```python
from build123d import *

# Parameters (mm, degrees)
F1_DEPTH = 150
F2_R     = 10
F4_W     = 30
F4_H     = 20
F5_DEPTH = 25
F6_R     = 7.5
F7_DEPTH = 10
F8_DEPTH = 25


with BuildPart() as f1:
    # F0 (on Top) → F1 (new body)
    with BuildSketch(Plane.XY):
        Polygon((0, 50), (-47.5528258148, 15.4508497187), (-29.3892626146, -40.4508497187), (29.3892626146, -40.4508497187), (47.5528258148, 15.4508497187), align=None)
    extrude(amount=F1_DEPTH)

    # F2
    f2_edges = [f1.edges().sort_by_distance(p)[0] for p in [
        (-29.389263, -40.45085, 75),
        (-47.552826, 15.45085, 75),
        (0, 50, 75),
        (47.552826, 15.45085, 75),
        (29.389263, -40.45085, 75),
    ]]
    fillet(f2_edges, radius=F2_R)

    # F4 (on face) → F5 (cut)
    with BuildSketch(Plane.XY.offset(150)):
        Rectangle(F4_W, F4_H)
    extrude(amount=-F5_DEPTH, mode=Mode.SUBTRACT)

    # F6 (on face) → F7 (cut)
    with BuildSketch(Plane.XZ.offset(40.4508497187)):
        with Locations((0, 129)):
            Circle(F6_R)
    extrude(amount=-F7_DEPTH, mode=Mode.SUBTRACT)

    # F8 (add): a face of the model
    f8_faces = [f1.faces().sort_by_distance(p)[0] for p in [
        (0, -40.4508497187, 73.5229190756),
    ]]
    extrude(f8_faces, amount=F8_DEPTH)


solid = f1.part
```
Input: part model. Units: mm. Frame: model coordinates. A direction names the side the tool comes from. Round coordinates to 2 decimals unless told otherwise and drop trailing zeros. Order: outer loops, then holes, each group sorted by start corner. A loop starts at its lowest first (then second) coordinate and runs counter-clockwise, first axis right, second up. Notation, with made-up numbers: (30, -39) - (49, -39) arc R27 cw to (49, -19) - close; hole circle Ø2 at (22, 14.25). An arc over 180 degrees is marked (long way). Answer in a Markdown table with one row per item.
Item 1: Line query: line 1 (X direction, y = -52, z = 90); line 2 (Y direction, x = -0.5, z = 12); line 3 (Y direction, x = 14.5, z = 142). Output: solid intervals per line, ascending.
Model answer:
| item | result |
|---|---|
| line 1 | x = -22.12 to 22.12 |
| line 2 | y = -65.45 to 47.63 |
| line 3 | y = -65.45 to -10, 10 to 39.47 |
Item 2: Pin query (flat end, axial travel): pin 1 (3 mm diameter, centred on y = -7.5, z = 65.5, fed in from -X); pin 2 (9 mm diameter, centred on x = 0, z = 129, fed in from -Y); pin 3 (6 mm diameter, centred on y = -49, z = 66, fed in from +X); pin 4 (10 mm diameter, centred on x = -25, y = 18, fed in from -Z). Return the tip coordinate at first contact, or that it passes through.
Model answer:
| item | result |
|---|---|
| pin 1 | stops at x = -40.58 |
| pin 2 | stops at y = -30.45 |
| pin 3 | stops at x = 22.12 |
| pin 4 | stops at z = 0 |
Item 3: Section query C-C (z = 65). Return the cut outline in (x, y).
Model answer:
| item | result |
|---|---|
| outline | (-45.31, 8.54) - (-31.63, -33.54) arc R10 ccw to (-22.12, -40.45) - (-22.12, -65.45) - (22.12, -65.45) - (22.12, -40.45) arc R10 ccw to (31.63, -33.54) - (45.31, 8.54) arc R10 ccw to (41.67, 19.72) - (5.88, 45.73) arc R10 ccw to (-5.88, 45.73) - (-41.67, 19.72) arc R10 ccw to start |
Item 4: Section query A-A (z = 129). Return the cut outline in (x, y).
Model answer:
| item | result |
|---|---|
| outline | (-45.31, 8.54) - (-31.63, -33.54) arc R10 ccw to (-22.12, -40.45) - (-22.12, -65.45) - (-7.5, -65.45) - (-7.5, -30.45) - (7.5, -30.45) - (7.5, -65.45) - (22.12, -65.45) - (22.12, -40.45) arc R10 ccw to (31.63, -33.54) - (45.31, 8.54) arc R10 ccw to (41.67, 19.72) - (5.88, 45.73) arc R10 ccw to (-5.88, 45.73) - (-41.67, 19.72) arc R10 ccw to start; hole (-15, -10) - (15, -10) - (15, 10) - (-15, 10) - close |
Item 5: Reachability of faces 5 (the flat face through (0, -65.451, 74)), 6 (the flat face through (-22.124, -53, 74)), 7 (the flat face through (0, -30.451, 129)), 8 (the flat face through (0, 0, 125)) from +Z, -Z, +X, -X, +Y, -Y: full face, straight path, thin tool, end or side. Return the list, or none.
Model answer:
| item | result |
|---|---|
| face 5 | +Z, -Z, +X, -X, -Y |
| face 6 | +Z, -Z, -X, -Y |
| face 7 | -Y |
| face 8 | +Z |
Item 6: Mould query, pull axis X, two halves, no side actions, for faces 1 (the flat face through (0, 10, 138)), 2 (the flat face through (-1, -8, 0)), 3 (the cylindrical face through (-0.976, -47.706, 136.436)), 4 (the flat face through (22.124, -53, 74)). Classes: released by +X, released by -X, zero draft, split by the parting line, or undercut.
Model answer:
| item | result |
|---|---|
| face 1 | undercut |
| face 2 | zero draft |
| face 3 | undercut |
| face 4 | released by +X |
Item 7: Section query D-D (y = 22). Return the cut outline in (x, z), then the cut area to 3 significant figures.
Model answer:
| item | result |
|---|---|
| outline | (-38.54, 0) - (38.54, 0) - (38.54, 150) - (-38.54, 150) - close |
| area | 11,600 mm² |
Item 8: Section query B-B (x = 0). Return the cut outline in (y, z).
Model answer:
| item | result |
|---|---|
| outline | (-65.45, 0) - (47.64, 0) - (47.64, 150) - (10, 150) - (10, 125) - (-10, 125) - (-10, 150) - (-65.45, 150) - (-65.45, 136.5) - (-30.45, 136.5) - (-30.45, 121.5) - (-65.45, 121.5) - close |
